```python
from build123d import *

# Parameters (mm, degrees)
F0_W      = 44.656470418
F0_H      = 33.8078811765
F1_DEPTH  = 16
F2_DEPTH  = 796
F3_DEPTH  = 196
F4_W      = 68.9578056335
F4_H      = 493.6993122101
F5_DEPTH  = 7
F6_DEPTH  = 9.7
F7_DEPTH  = 99.33
F8_DEPTH  = 99.33
F9_DEPTH  = 17.34
F10_DEPTH = 102.97
F11_W     = 35.2807044983
F11_H     = 492.0964837074
F12_DEPTH = 7
F13_DEPTH = 37.27
F14_DEPTH = 6.58
F15_DEPTH = 106.63
F16_DEPTH = 5.87
F17_DEPTH = 200
F18_DEPTH = 200
F19_DEPTH = 200
F20_DEPTH = 200
F21_DEPTH = 200
F22_DEPTH = 200
F23_DEPTH = 600
F24_DEPTH = 600
F25_DEPTH = 600
F26_DEPTH = 200
F27_DEPTH = 200
F28_DEPTH = 200
F29_DEPTH = 200
F30_DEPTH = 200
F31_DEPTH = 200
F32_DEPTH = 200
F33_DEPTH = 200
F34_DEPTH = 200
F35_DEPTH = 200
F36_DEPTH = 200
F37_DEPTH = 200
F38_R     = 3


with BuildPart() as f1:
    # F0 (on Front) → F1 (new body)
    with BuildSketch(Plane.XZ):
        with Locations((22.328235209, 16.9039405882)):
            Rectangle(F0_W, F0_H)
    extrude(amount=F1_DEPTH)

    # F2 (add): a face of the model
    f2_faces = [f1.faces().sort_by_distance(p)[0] for p in [
        (22.328235209, -8, 0),
    ]]
    extrude(f2_faces, amount=-F2_DEPTH)

    # F3 (add): a face of the model
    f3_faces = [f1.faces().sort_by_distance(p)[0] for p in [
        (0, -8, 398),
    ]]
    extrude(f3_faces, amount=-F3_DEPTH)

    # F4 (on face) → F5 (cut)
    with BuildSketch(Plane.XZ.offset(16)):
        with Locations((94.1769480705, 399.8196721077)):
            Rectangle(F4_W, F4_H)
    extrude(amount=-F5_DEPTH, mode=Mode.SUBTRACT)

    # F6 (cut): a face of the model
    f6_faces = [f1.faces().sort_by_distance(p)[0] for p in [
        (59.6980452538, -12.5, 399.8196721077),
    ]]
    extrude(f6_faces, amount=-F6_DEPTH, mode=Mode.SUBTRACT)

    # F7 (add): a face of the model
    f7_faces = [f1.faces().sort_by_distance(p)[0] for p in [
        (89.3269480705, -12.5, 646.6693282127),
    ]]
    extrude(f7_faces, amount=-F7_DEPTH)

    # F8 (cut): a face of the model
    f8_faces = [f1.faces().sort_by_distance(p)[0] for p in [
        (89.3269480705, -12.5, 646.6693282127),
    ]]
    extrude(f8_faces, amount=-F8_DEPTH, mode=Mode.SUBTRACT)

    # F9 (cut): a face of the model
    f9_faces = [f1.faces().sort_by_distance(p)[0] for p in [
        (128.6558508873, -12.5, 449.4846721077),
    ]]
    extrude(f9_faces, amount=-F9_DEPTH, mode=Mode.SUBTRACT)

    # F10 (cut): a face of the model
    f10_faces = [f1.faces().sort_by_distance(p)[0] for p in [
        (97.9969480705, -12.5, 152.9700160027),
    ]]
    extrude(f10_faces, amount=-F10_DEPTH, mode=Mode.SUBTRACT)

    # F11 (on face) → F12 (join)
    with BuildSketch(Plane.XZ.offset(9)):
        with Locations((91.7714834213, 432.6795041561)):
            Rectangle(F11_W, F11_H)
    extrude(amount=F12_DEPTH)

    # F13 (add): a face of the model
    f13_faces = [f1.faces().sort_by_distance(p)[0] for p in [
        (91.7714834213, -12.5, 678.7277460098),
    ]]
    extrude(f13_faces, amount=F13_DEPTH)

    # F14 (add): a face of the model
    f14_faces = [f1.faces().sort_by_distance(p)[0] for p in [
        (109.4118356705, -12.5, 451.3145041561),
    ]]
    extrude(f14_faces, amount=F14_DEPTH)

    # F15 (add): a face of the model
    f15_faces = [f1.faces().sort_by_distance(p)[0] for p in [
        (95.0614834213, -12.5, 186.6312623024),
    ]]
    extrude(f15_faces, amount=F15_DEPTH)

    # F16 (cut): a face of the model
    f16_faces = [f1.faces().sort_by_distance(p)[0] for p in [
        (74.1311311722, -12.5, 397.9995041561),
    ]]
    extrude(f16_faces, amount=-F16_DEPTH, mode=Mode.SUBTRACT)

    # F17 (add): a face of the model
    f17_faces = [f1.faces().sort_by_distance(p)[0] for p in [
        (196, -8, 398),
    ]]
    extrude(f17_faces, amount=F17_DEPTH)

    # F18 (cut): a face of the model
    f18_faces = [f1.faces().sort_by_distance(p)[0] for p in [
        (145.9958508873, -12.5, 397.9996721077),
    ]]
    extrude(f18_faces, amount=-F18_DEPTH, mode=Mode.SUBTRACT)

    # F19 (add): a face of the model
    f19_faces = [f1.faces().sort_by_distance(p)[0] for p in [
        (115.9918356705, -12.5, 397.9995041561),
    ]]
    extrude(f19_faces, amount=F19_DEPTH)

    # F20 (add): a face of the model
    f20_faces = [f1.faces().sort_by_distance(p)[0] for p in [
        (396, -8, 398),
    ]]
    extrude(f20_faces, amount=F20_DEPTH)

    # F21 (cut): a face of the model
    f21_faces = [f1.faces().sort_by_distance(p)[0] for p in [
        (345.9958508873, -12.5, 397.9996721077),
    ]]
    extrude(f21_faces, amount=-F21_DEPTH, mode=Mode.SUBTRACT)

    # F22 (add): a face of the model
    f22_faces = [f1.faces().sort_by_distance(p)[0] for p in [
        (315.9918356705, -12.5, 397.9995041561),
    ]]
    extrude(f22_faces, amount=F22_DEPTH)

    # F23 (cut): a face of the model
    f23_faces = [f1.faces().sort_by_distance(p)[0] for p in [
        (297.9964834213, -12.5, 80.0012623024),
    ]]
    extrude(f23_faces, amount=-F23_DEPTH, mode=Mode.SUBTRACT)

    # F24 (add): a face of the model
    f24_faces = [f1.faces().sort_by_distance(p)[0] for p in [
        (297.9969480705, -12.5, 50.0000160027),
    ]]
    extrude(f24_faces, amount=F24_DEPTH)

    # F25 (cut): a face of the model
    f25_faces = [f1.faces().sort_by_distance(p)[0] for p in [
        (298, -8, 0),
    ]]
    extrude(f25_faces, amount=-F25_DEPTH, mode=Mode.SUBTRACT)

    # F26 (add): a face of the model
    f26_faces = [f1.faces().sort_by_distance(p)[0] for p in [
        (298, -8, 600),
    ]]
    extrude(f26_faces, amount=F26_DEPTH)

    # F27 (cut): a face of the model
    f27_faces = [f1.faces().sort_by_distance(p)[0] for p in [
        (297.9969480705, -12.5, 650.0000160027),
    ]]
    extrude(f27_faces, amount=-F27_DEPTH, mode=Mode.SUBTRACT)

    # F28 (add): a face of the model
    f28_faces = [f1.faces().sort_by_distance(p)[0] for p in [
        (297.9964834213, -12.5, 680.0012623024),
    ]]
    extrude(f28_faces, amount=F28_DEPTH)

    # F29 (add): a face of the model
    f29_faces = [f1.faces().sort_by_distance(p)[0] for p in [
        (596, -8, 598),
    ]]
    extrude(f29_faces, amount=F29_DEPTH)

    # F30 (cut): a face of the model
    f30_faces = [f1.faces().sort_by_distance(p)[0] for p in [
        (545.9958508873, -12.5, 597.9996721077),
    ]]
    extrude(f30_faces, amount=-F30_DEPTH, mode=Mode.SUBTRACT)

    # F31 (add): a face of the model
    f31_faces = [f1.faces().sort_by_distance(p)[0] for p in [
        (515.9918356705, -12.5, 597.9995041561),
    ]]
    extrude(f31_faces, amount=F31_DEPTH)

    # F32 (cut): a face of the model
    f32_faces = [f1.faces().sort_by_distance(p)[0] for p in [
        (397.9964834213, -12.5, 480.0012623024),
    ]]
    extrude(f32_faces, amount=-F32_DEPTH, mode=Mode.SUBTRACT)

    # F33 (add): a face of the model
    f33_faces = [f1.faces().sort_by_distance(p)[0] for p in [
        (397.9969480705, -12.5, 450.0000160027),
    ]]
    extrude(f33_faces, amount=F33_DEPTH)

    # F34 (cut): a face of the model
    f34_faces = [f1.faces().sort_by_distance(p)[0] for p in [
        (398, -8, 400),
    ]]
    extrude(f34_faces, amount=-F34_DEPTH, mode=Mode.SUBTRACT)

    # F35 (add): a face of the model
    f35_faces = [f1.faces().sort_by_distance(p)[0] for p in [
        (398, -8, 600),
    ]]
    extrude(f35_faces, amount=F35_DEPTH)

    # F36 (cut): a face of the model
    f36_faces = [f1.faces().sort_by_distance(p)[0] for p in [
        (397.9969480705, -12.5, 650.0000160027),
    ]]
    extrude(f36_faces, amount=-F36_DEPTH, mode=Mode.SUBTRACT)

    # F37 (add): a face of the model
    f37_faces = [f1.faces().sort_by_distance(p)[0] for p in [
        (397.9964834213, -12.5, 680.0012623024),
    ]]
    extrude(f37_faces, amount=F37_DEPTH)

    # F38
    f38_edges = [f1.edges().sort_by_distance(p)[0] for p in [
        (397.996483, -16, 715.997746),
        (715.991836, -16, 597.999504),
        (397.996483, -16, 480.001262),
        (80.001131, -16, 597.999504),
        (0, -16, 598),
        (398, -16, 400),
        (796, -16, 598),
        (398, -16, 796),
        (49.998045, -16, 597.999672),
        (397.996948, -16, 745.999328),
        (745.995851, -16, 597.999672),
        (397.996948, -16, 450.000016),
    ]]
    fillet(f38_edges, radius=F38_R)


solid = f1.part
```
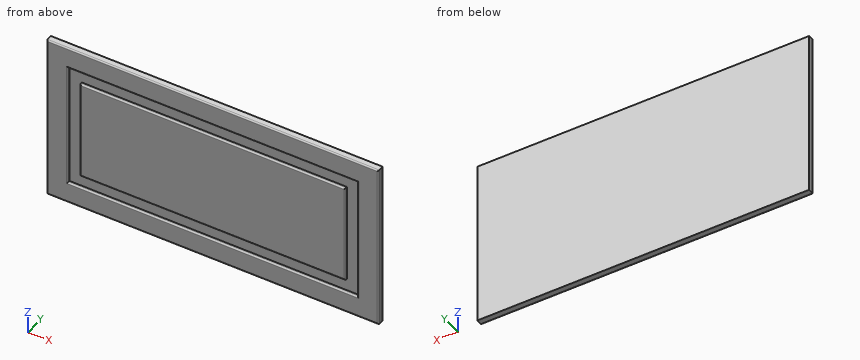
Could you check a few things on this model? Use its own coordinates, in mm. Round coordinates to 2 decimals unless told otherwise and drop trailing zeros. Loops run counter-clockwise (first coordinate to the right, second up) from the corner with the lowest first, then second, coordinate; pieces in that order, holes last. Notation, with made-up numbers: M 75,70.5 L 108,70.5 A15 ccw 108,86.5 Z; hole C 67.25,9.25 d10. An arc over 180 degrees is marked long. Put each result on its own line as item: value.
Q1. Imagine slicing it at B-B (x = 494.5). Write out the boundary of the cut face in (y, z), then the cut area to 3 significant figures.
Check result:
outline: M -16,403 A3 ccw -13,400 L 0,400 L 0,796 L -13,796 A3 ccw -16,793 L -16,749 A3 ccw -13,746 L -9,746 L -9,716 L -13,716 A3 ccw -16,713 L -16,483 A3 ccw -13,480 L -9,480 L -9,450 L -13,450 A3 ccw -16,447 Z
area: 5,900 mm2
Q2. Imagine slicing it at C-C (z = 657). Write out the boundary of the cut face in (x, y).
Check result:
outline: M 0,-13 A3 ccw 3,-16 L 47,-16 A3 ccw 50,-13 L 50,-9 L 80,-9 L 80,-13 A3 ccw 83,-16 L 712.99,-16 A3 ccw 715.99,-13 L 715.99,-9 L 746,-9 L 746,-13 A3 ccw 749,-16 L 793,-16 A3 ccw 796,-13 L 796,0 L 0,0 Z
Q3. I need wall thicknesses on probe 1 along X at (y, z) = (-12.25, 691); probe 2 along Z at (x, y) = (292.5, -13); probe 3 along Y at (x, z) = (724.5, 703.5). Which ranges of each line are inside material? Lowest first, please.
Check result:
probe 1: 0 to 50, 80 to 715.99, 746 to 796
probe 2: 400 to 450, 480 to 716, 746 to 796
probe 3: -9 to 0
Q4. Imagine slicing it at A-A (z = 728.5). Write out the boundary of the cut face in (x, y), then the cut area to 3 significant figures.
Check result:
outline: M 0,-13 A3 ccw 3,-16 L 47,-16 A3 ccw 50,-13 L 50,-9 L 746,-9 L 746,-13 A3 ccw 749,-16 L 793,-16 A3 ccw 796,-13 L 796,0 L 0,0 Z
area: 7,860 mm2
